```python
from build123d import *

# Parameters (mm, degrees)
SKETCH2_W               = 47.3
SKETCH2_H               = 24.9
BOSS_EXTRUDE1_DEPTH     = 14.3
CUT_EXTRUDE1_DEPTH      = 38.199764784
CUT_EXTRUDE1_DEPTH_BACK = 38.199764784
FILLET1_R               = 1


with BuildPart() as part:
    # Sketch2 → Boss-Extrude1 (new body)
    with BuildSketch(Plane(origin=(0, 0, 0), x_dir=(1, 0, 0), z_dir=(0, 1, 0))):
        Rectangle(SKETCH2_W, SKETCH2_H)
    extrude(amount=-BOSS_EXTRUDE1_DEPTH)

    # Sketch3 → Cut-Extrude1 (cut, two sides: drawn at the far end of the back side and taken through both)
    with BuildSketch(Plane(origin=(0, 0, -12.45), x_dir=(-1, 0, 0), z_dir=(0, 0, -1)).offset(-CUT_EXTRUDE1_DEPTH_BACK)):
        with BuildLine():
            Line((-23.65, -4.326263992), (-4.128269017, -4.326263992))
            add(Edge.make_bspline(
                [(-4.128269017, -4.326263992), (1.486176846, -4.326263992), (6.258882745, 0), (12.779413221, 0)],
                knots=[0, 0, 0, 0, 1, 1, 1, 1], degree=3))
            Line((12.779413221, 0), (-23.65, 0))
            Line((-23.65, 0), (-23.65, -4.326263992))
        make_face()
    extrude(amount=CUT_EXTRUDE1_DEPTH + CUT_EXTRUDE1_DEPTH_BACK, mode=Mode.SUBTRACT)

    # Fillet1
    fillet1_edges = [part.edges().sort_by_distance(p)[0] for p in [
        (-23.65, -14.3, 0),
        (-23.65, 0, 0),
        (-18.214706611, 0, -12.45),
        (-23.65, -7.15, -12.45),
        (0, -14.3, -12.45),
        (13.889134509, -4.326263992, -12.45),
        (-4.294045932, -2.040368807, -12.45),
        (23.65, -9.313131996, -12.45),
        (23.65, -14.3, 0),
        (23.65, -4.326263992, 0),
        (13.889134509, -4.326263992, 12.45),
        (23.65, -9.313131996, 12.45),
        (0, -14.3, 12.45),
        (-23.65, -7.15, 12.45),
        (-18.214706611, 0, 12.45),
        (-4.294045921, -2.040368812, 12.45),
    ]]
    fillet(fillet1_edges, radius=FILLET1_R)


solid = part.part
```
Geometry: final body of the model. Coordinates: model frame, mm. A direction names the side the tool comes from. Coordinates: 2 decimals unless noted, no trailing zeros. Order: outer loops, then holes, each group sorted by start corner. A loop starts at its lowest first (then second) coordinate and runs counter-clockwise, first axis right, second up.
Item 1: Access query for faces 1 (the face through (14, -4.326, 0)), 2 (the face through (13.259, -4.627, 12.165)), 3 (the face through (13.519, -4.627, -12.165)). Directions: +Z, -Z, +X, -X, +Y, -Y. A direction counts if a zero-diameter tool reaches every point of the face in a straight line with its end or side. Return the directions, or none.
Answer:
face 1: +Z, -Z, +X, +Y
face 2: +Z, +X, +Y
face 3: -Z, +X, +Y
Item 2: Contact query for flat-ended pins moving along their axis: P1, Ø10, axis at x = -12, z = -6.5, coming from the +Y side; P2, Ø1.5, axis at x = 8, z = 3, coming from the +Y side. Output: stop coordinate, or through.
Answer:
P1: stops at y = 0
P2: stops at y = -4.33
Item 3: Section query A-A (x = 5.5). Output: boundary loops of the cut face in (y, z).
Answer:
outline: (-14.3, -11.45) arc R1 ccw to (-13.3, -12.45) - (-5.33, -12.45) arc R1 ccw to (-4.33, -11.45) - (-4.33, 11.45) arc R1 ccw to (-5.33, 12.45) - (-13.3, 12.45) arc R1 ccw to (-14.3, 11.45) - close
Item 4: Material intervals for line 1 along Y through (x, z) = (7, -2); line 2 along Z through (x, y) = (19, -5.25); line 3 along Y through (x, z) = (-1, 1), sorted ascending.
Answer:
line 1: y = -14.3 to -4.33
line 2: z = -12.45 to 12.45
line 3: y = -14.3 to -3.31
